from build123d import *

# Parameters (mm, degrees)
SKETCH_1_R      = 2.1
EXTRUDE_1_DEPTH = 3


with BuildPart() as part:
    # 草图1 → 凸台-拉伸1 (new body)
    with BuildSketch(Plane(origin=(0, 0, 0), x_dir=(0, 0, -1), z_dir=(1, 0, 0))):
        with BuildLine():
            Line((59.529555332, 44.185221984), (59.529555332, 25.226213997))
            ThreePointArc((59.529555332, 25.226213997), (58.943993255, 23.142560073), (57.358748495, 21.668960509))
            Line((57.358748495, 21.668960509), (16.843911029, 0.835622672))
            ThreePointArc((16.843911029, 0.835622672), (13.51321063, -0.403694355), (9.984436669, -0.82467675))
            Line((9.984436669, -0.82467675), (-12.543438126, -0.82467675))
            ThreePointArc((-12.543438126, -0.82467675), (-15.441612868, -0.542033278), (-18.230567587, 0.295245495))
            Line((-18.230567587, 0.295245495), (-39.640671861, 9.067677244))
            ThreePointArc((-39.640671861, 9.067677244), (-41.445720436, 10.540385022), (-42.124104005, 12.769031312))
            Line((-42.124104005, 12.769031312), (-42.124104005, 44.185221984))
            ThreePointArc((-42.124104005, 44.185221984), (-40.95253113, 47.013649109), (-38.124104005, 48.185221984))
            Line((-38.124104005, 48.185221984), (-2.92315645, 48.185221984))
            Line((-2.92315645, 48.185221984), (55.529555332, 48.185221984))
            ThreePointArc((55.529555332, 48.185221984), (58.357982457, 47.013649109), (59.529555332, 44.185221984))
        make_face()
        with Locations((40.626001942, 41.835221984)):
            Circle(SKETCH_1_R, mode=Mode.SUBTRACT)
        with Locations((-35.573998058, 15.266821984)):
            Circle(SKETCH_1_R, mode=Mode.SUBTRACT)
        with Locations((-22.873998058, 15.266821984)):
            Circle(SKETCH_1_R, mode=Mode.SUBTRACT)
        with Locations((-10.173998058, 15.266821984)):
            Circle(SKETCH_1_R, mode=Mode.SUBTRACT)
        with Locations((2.526001942, 15.266821984)):
            Circle(SKETCH_1_R, mode=Mode.SUBTRACT)
        with Locations((15.226001942, 15.266821984)):
            Circle(SKETCH_1_R, mode=Mode.SUBTRACT)
        with Locations((27.926001942, 15.266821984)):
            Circle(SKETCH_1_R, mode=Mode.SUBTRACT)
        with Locations((53.326001942, 41.835221984)):
            Circle(SKETCH_1_R, mode=Mode.SUBTRACT)
        with Locations((53.326001942, 29.135221984)):
            Circle(SKETCH_1_R, mode=Mode.SUBTRACT)
        with Locations((40.626001942, 29.135221984)):
            Circle(SKETCH_1_R, mode=Mode.SUBTRACT)
        with Locations((-35.573998058, 41.835221984)):
            Circle(SKETCH_1_R, mode=Mode.SUBTRACT)
        with Locations((-35.573998058, 29.135221984)):
            Circle(SKETCH_1_R, mode=Mode.SUBTRACT)
        with Locations((27.926001942, 41.835221984)):
            Circle(SKETCH_1_R, mode=Mode.SUBTRACT)
        with Locations((27.926001942, 29.135221984)):
            Circle(SKETCH_1_R, mode=Mode.SUBTRACT)
    extrude(amount=EXTRUDE_1_DEPTH)


solid = part.part
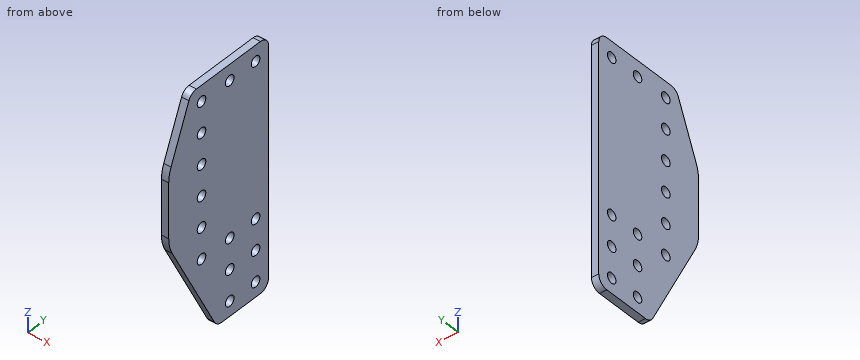
Verification items for the finished model (mm, model axes). Give positions to 0.01 mm unless a question says otherwise; leave off trailing zeros. Loops run counter-clockwise (first coordinate to the right, second up) from the corner with the lowest first, then second, coordinate; pieces in that order, holes last. Notation, with made-up numbers: (-18.75, 53.25) - (-1.75, 53.25) arc R35 cw to (-1.75, 89.25) - close; hole circle Ø1 at (88.5, 75). An arc over 180 degrees is marked (long way). Write each question's results on one line, items separated by ' | '.
1) Material ranges on L1, parallel to Y at x = 2.5, z = -51.5; L2, parallel to Y at x = 1.2, z = 35.5; L3, parallel to Y at x = 0.2, z = 13, recorded low to high. Write a range as from..to.
Solution:
L1: 18.66..28.1, 30.17..40.8, 42.87..48.19 | L2: 7.37..13.17, 17.37..27.04, 31.23..39.74, 43.93..48.19 | L3: -0.82..48.19
2) Sectioned sample at D-D on y = 7. Record the boundary of the cut face in (x, z), plus the area to 3 significant figures.
Solution:
outline: (0, -28.83) - (3, -28.83) - (3, 34.59) - (0, 34.59) - close | area: 190 mm2
3) Sectioned sample at B-B on x = 0.85. Count the separate pieces of the cut face and the enclosed holes in it, plus the area to 3 significant figures.
Solution:
separate pieces: 1 | enclosed holes: 14 | area: 4,090 mm2
4) Sectioned sample at C-C on z = 35.5. Record the boundary of the cut face in (x, y), plus the area to 3 significant figures.
Solution:
outline: (0, 7.37) - (3, 7.37) - (3, 13.17) - (0, 13.17) - close; (0, 17.37) - (3, 17.37) - (3, 27.04) - (0, 27.04) - close; (0, 31.23) - (3, 31.23) - (3, 39.74) - (0, 39.74) - close; (0, 43.93) - (3, 43.93) - (3, 48.19) - (0, 48.19) - close | area: 84.7 mm2
5) Depth check by flat-ended pin: P1, Ø2.5, axis at y = 41.84, z = 35.57, coming from the +X side. Enter the tip coordinate at first touch or a pass-through.
Solution:
P1: through
6) Sectioned sample at A-A on z = -28. Record the boundary of the cut face in (x, y), plus the area to 3 significant figures.
Solution:
outline: (0, 6.57) - (3, 6.57) - (3, 13.17) - (0, 13.17) - close; (0, 17.37) - (3, 17.37) - (3, 27.04) - (0, 27.04) - close; (0, 31.23) - (3, 31.23) - (3, 39.74) - (0, 39.74) - close; (0, 43.93) - (3, 43.93) - (3, 48.19) - (0, 48.19) - close | area: 87.1 mm2
